from build123d import *

# Parameters (mm, degrees)
SKETCH_2_R               = 4
CUT_EXTRUDE_1_DEPTH      = 49.744230428
CUT_EXTRUDE_START        = -8
SKETCH_3_R               = 8
CUT_EXTRUDE_2_DEPTH      = 8
CHAMFER_1_SIZE2          = 2.309401077
CHAMFER_1_SIZE           = 4
HOLE_WIZARD_M5_1_D       = 4.2
CUT_EXTRUDE_3_DEPTH      = 48.339201514
PATTERN_CIRCULAR_1_COUNT = 3
CHAMFER_4_SIZE           = 0.5
EXTRUDE_START            = 15
EXTRUDE_1_DEPTH          = 15
CHAMFER_5_SIZE           = 1.5
CHAMFER_6_SIZE           = 0.5
FILLET_1_R               = 0.2


# Some blends are built 0.0001 mm under size
with BuildPart() as part:
    # 草图1 → 旋转1 (revolve)
    with BuildSketch(Plane.XY, mode=Mode.PRIVATE) as revolve_1_sk:
        Polygon((0, 0), (0, 10), (3, 10), (3, 30), (8, 30), (8, 9.6), (10.8, 9.6), (10.8, 8.5), (21, 8.5), (21, 8), (22, 8), (22, 8.5), (24, 8.5), (24, 0), align=None)
    revolve(revolve_1_sk.sketch.rotate(Axis((24, 0, 0), (-1, 0, 0)), 90), axis=Axis((24, 0, 0), (-1, 0, 0)))

    # 草图2 → 切除-拉伸1 (cut, through all)
    with BuildSketch(Plane(origin=(24, 0, 0), x_dir=(0, 0, -1), z_dir=(1, 0, 0))):
        Circle(SKETCH_2_R)
    extrude(amount=-CUT_EXTRUDE_1_DEPTH, mode=Mode.SUBTRACT)

    # 草图3 → 切除-拉伸2 (cut)
    with BuildSketch(Plane.ZY.offset(CUT_EXTRUDE_START)):
        with Locations(Location((0, 0, 0), (0, 0, 180))):
            Circle(SKETCH_3_R)
    extrude(amount=CUT_EXTRUDE_2_DEPTH, mode=Mode.SUBTRACT)

    # 倒角1
    chamfer_1_edges = [part.edges().sort_by_distance(p)[0] for p in [
        (8, 0, 4),
    ]]
    chamfer_1_side = [part.faces().sort_by_distance(p)[0] for p in [
        (8, 0, 4.046188022),
    ]]
    chamfer(chamfer_1_edges, length=CHAMFER_1_SIZE - 0.0001, length2=CHAMFER_1_SIZE2 - 0.0001, reference=chamfer_1_side[0])  # a hair under: the kernel refuses the full size

    # M5 螺纹孔1 (through all)
    with Locations(Plane(origin=(3, 25, 0), x_dir=(0, 0, -1), z_dir=(-1, 0, 0))):
        with Locations((0, 0), (-21.650635095, 37.5), (21.650635095, 37.5)):
            Hole(HOLE_WIZARD_M5_1_D / 2)

    # 草图4 → 切除-拉伸3 (cut, through all)
    with BuildSketch(Plane.ZY.offset(-3)):
        with BuildLine():
            ThreePointArc((-27.710194429, -21.380952381), (0, -35), (27.710194429, -21.380952381))
            ThreePointArc((27.710194429, -21.380952381), (0, -13), (-27.710194429, -21.380952381))
        make_face()
    cut_extrude_3 = extrude(amount=-CUT_EXTRUDE_3_DEPTH, mode=Mode.SUBTRACT)

    # 阵列(圆周)1: 切除-拉伸3 ×3 about axis
    pattern_circular_1_axis = Axis((0, 0, 0), (1, 0, 0))
    for i in range(1, PATTERN_CIRCULAR_1_COUNT):
        add(cut_extrude_3.rotate(pattern_circular_1_axis, i * 360 / PATTERN_CIRCULAR_1_COUNT), mode=Mode.SUBTRACT)

    # 倒角2
    # the kernel refuses this chamfer: 1.262336382, 1 mm, written as the material it takes off along each edge
    with BuildSketch(Plane(origin=(-0.323534522, -18.801587302, -23.377346191), x_dir=(0, 0.7894182220381707, -0.6138557409637001), z_dir=(1, 0, 0)), Plane(origin=(-0.323534522, -10.844582024, 27.97132533), x_dir=(0, -0.9263237769525716, -0.3767283640135453), z_dir=(1, 0, 0)), Plane(origin=(-0.323534522, 29.646169325, -4.593979139), x_dir=(0, 0.13690555491440626, 0.9905841049772496), z_dir=(1, 0, 0))) as chamfer_2_piece_1:
        with BuildLine():
            Line((0.983994902, 0), (-0.239625676, 1.264429883))
            ThreePointArc((-0.239625676, 1.264429883), (-0.119678092, 0.653717986), (0, 0))
            ThreePointArc((0, 0), (0.509546154, -0.004029497), (0.983994902, 0))
        make_face()
    extrude(amount=11.647069044, mode=Mode.SUBTRACT)
    with BuildSketch(Plane(origin=(-0.323534522, -10.844582024, -27.97132533), x_dir=(0, 0.5426204152715339, 0.8399780264569711), z_dir=(1, 0, 0)), Plane(origin=(-0.323534522, 29.646169325, 4.593979139), x_dir=(0, -0.9987525171682211, 0.04993405100872917), z_dir=(1, 0, 0))) as chamfer_2_piece_2:
        with BuildLine():
            Line((1.28693566, 0), (-0.183218517, 0.966786917))
            ThreePointArc((-0.183218517, 0.966786917), (-0.098835833, 0.499884984), (0, 0))
            ThreePointArc((0, 0), (0.664569743, 0.004136227), (1.28693566, 0))
        make_face()
    extrude(amount=11.647069044, mode=Mode.SUBTRACT)
    with BuildSketch(Plane(origin=(-0.323534522, -18.801587302, 23.377346191), x_dir=(0, 0.7894182220381672, 0.6138557409637047), z_dir=(1, 0, 0))) as chamfer_2_piece_3:
        with BuildLine():
            Line((0.983994902, 0), (-0.239625676, -1.264429883))
            ThreePointArc((-0.239625676, -1.264429883), (-0.119678092, -0.653717986), (0, 0))
            ThreePointArc((0, 0), (0.509546154, 0.004029497), (0.983994902, 0))
        make_face()
    extrude(amount=11.647069044, mode=Mode.SUBTRACT)

    # 倒角4
    chamfer_4_edges = [part.edges().sort_by_distance(p)[0] for p in [
        (0, 0, 10),
    ]]
    chamfer(chamfer_4_edges, length=CHAMFER_4_SIZE)

    # 草图7 → 凸台-拉伸1 (add)
    with BuildSketch(Plane(origin=(24, 0, 0), x_dir=(0, 0, -1), z_dir=(1, 0, 0)).offset(EXTRUDE_START)):
        with BuildLine():
            Line((-6.7, -6), (6.7, -6))
            Line((6.7, -6), (6.7, 3.708099244))
            Line((6.7, 3.708099244), (1.5, 3.708099244))
            ThreePointArc((1.5, 3.708099244), (0, -4), (-1.5, 3.708099244))
            Line((-1.5, 3.708099244), (-6.7, 3.708099244))
            Line((-6.7, 3.708099244), (-6.7, -6))
        make_face()
    extrude(amount=-EXTRUDE_1_DEPTH)

    # 倒角5
    # the kernel refuses this chamfer: 1.5 mm, written as the material it takes off along each edge
    with BuildSketch(Plane(origin=(42.857524482, 3.708099244, 6.7), x_dir=(0, 0, -1), z_dir=(-1, 0, 0)), Plane(origin=(42.857524482, -6, 6.7), x_dir=(0, 1, 0), z_dir=(-1, 0, 0))) as chamfer_5_piece_1:
        Polygon((CHAMFER_5_SIZE, 0), (0, CHAMFER_5_SIZE), (0, 0), align=None)
    extrude(amount=18.857524482, mode=Mode.SUBTRACT)
    with BuildSketch(Plane(origin=(42.857524482, -6, -6.7), x_dir=(0, 1, 0), z_dir=(-1, 0, 0)), Plane(origin=(42.857524482, 3.708099244, -6.7), x_dir=(0, 0, 1), z_dir=(-1, 0, 0))) as chamfer_5_piece_2:
        Polygon((CHAMFER_5_SIZE, 0), (0, -CHAMFER_5_SIZE), (0, 0), align=None)
    extrude(amount=18.857524482, mode=Mode.SUBTRACT)

    # 倒角6
    chamfer_6_edges = [part.edges().sort_by_distance(p)[0] for p in [
        (39, -4, 0),
    ]]
    chamfer(chamfer_6_edges, length=CHAMFER_6_SIZE)

    # 圆角1
    # the kernel refuses this fillet: 0.2 mm, written as the material it takes off along each edge
    with BuildSketch(Plane(origin=(40.52345201, 3.708099244, 1.5), x_dir=(0, -0.464696875551773, 0.8854698266188521), z_dir=(-1, 0, 0))) as fillet_1_piece_1:
        with BuildLine():
            CenterArc((0.809621655, 0.199022765), FILLET_1_R, 117.690606121, 146.643100594)
            Line((0.71668228, 0.376116731), (0, 0))
            ThreePointArc((0, 0), (0.394937393, 0.019544692), (0.789874786, 0))
        make_face()
    extrude(amount=16.52345201, mode=Mode.SUBTRACT)
    with BuildSketch(Plane(origin=(40.52345201, 3.708099244, -1.5), x_dir=(0, -0.46469687555177314, -0.885469826618852), z_dir=(-1, 0, 0))) as fillet_1_piece_2:
        with BuildLine():
            CenterArc((0.809621655, -0.199022765), FILLET_1_R, 95.666293284, 146.643100594)
            Line((0.71668228, -0.376116731), (0, 0))
            ThreePointArc((0, 0), (0.394937393, -0.019544692), (0.789874786, 0))
        make_face()
    extrude(amount=16.52345201, mode=Mode.SUBTRACT)


solid = part.part
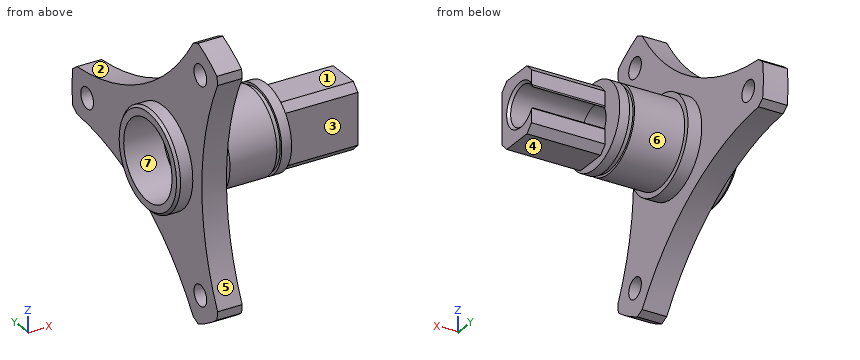
Geometry: final body of the model. Coordinates: model frame, mm. Face numbers are marked on the shaded views. A direction names the side the tool comes from. Give positions to 0.01 mm unless a question says otherwise; leave off trailing zeros. Loops run counter-clockwise (first coordinate to the right, second up) from the corner with the lowest first, then second, coordinate; pieces in that order, holes last. Notation, with made-up numbers: M 70,1.25 L 113,1.25 A20 cw 113,19.25 Z; hole C -39.75,23 d7. An arc over 180 degrees is marked long. Put each result on its own line as item: value.
1) Material intervals for L1, parallel to Y at x = 4, z = 0; L2, parallel to Z at x = 32.25, y = 0; L3, parallel to Z at x = 5.8, y = -12.5, sorted ascending. Write a range as from..to.
Computed values:
L1: y = -13..-8, 8..22.9, 27.1..30
L2: z = -6.7..-4, 4..6.7
L3: z = -27.27..-23.75, -19.55..19.55, 23.75..27.27
2) Cut plane A-A, the plane x = 5. Return the cut outline in (y, z), plus the area to 3 significant figures.
Computed values:
outline: M -18.21,-22.23 L -18.02,-23.98 A30 ccw -11.76,-27.6 L -10.15,-26.89 A50 cw 28.36,-4.66 L 29.78,-3.62 A30 ccw 29.78,3.62 L 28.36,4.66 A50 cw -10.15,26.89 L -11.76,27.6 A30 ccw -18.02,23.98 L -18.21,22.23 A50 cw Z; hole C -12.5,-21.65 d4.2; hole C -12.5,21.65 d4.2; hole C 0,0 d16; hole C 25,0 d4.2
area: 938 mm^2
3) First-contact query: P1, Ø1.5, axis at x = 4, y = 5.5, coming from the -Z side; P2, Ø12, axis at x = 11, z = -8, coming from the +Y side; P3, Ø5.5, axis at x = 30.5, y = -1.5, coming from the +Z side. Flat tips, straight axial feed; report the tip coordinate or a pass-through.
Computed values:
P1: stops at z = -12.32
P2: stops at y = 29.87
P3: stops at z = 6.7
4) Reachability of the marked faces 1, 2 and 3 from +Z, -Z, +X, -X, +Y, -Y: full face, straight path, thin tool, end or side. Return the list, or none.
Computed values:
face 1: +Z, +X, +Y, -Y
face 2: +Z, +X, -X, +Y
face 3: +Z, -Z, +X, -Y
5) Mould query, pull axis Z, two halves, no side actions, for the marked faces 4, 5, 6 and 7. Classes: released by +Z, released by -Z, zero draft, split by the parting line, or undercut.
Computed values:
face 4: released by -Z
face 5: undercut
face 6: split by the parting line
face 7: undercut
6) Cut plane C-C, the plane y = 25. Return the cut outline in (x, z), plus the area to 3 significant figures.
Computed values:
outline: M 3,-4.98 L 8,-4.98 L 8,-2.1 L 3,-2.1 Z; M 3,2.1 L 8,2.1 L 8,4.98 L 3,4.98 Z
area: 28.8 mm^2
7) Cut plane B-B, the plane z = 0. Give the number of separate pieces and of enclosed holes in the cut face, plus the area to 3 significant figures.
Computed values:
separate pieces: 3
enclosed holes: 0
area: 296 mm^2
8) Cut plane D-D, the plane x = 31. Return the cut outline in (y, z), plus the area to 3 significant figures.
Computed values:
outline: M -6,-5.2 L -4.5,-6.7 L 2.21,-6.7 L 3.71,-5.2 L 3.71,-2.31 A0.2 ccw 3.34,-2.2 A4 cw long 3.34,2.2 A0.2 ccw 3.71,2.31 L 3.71,5.2 L 2.21,6.7 L -4.5,6.7 L -6,5.2 Z
area: 75.7 mm^2
